The listing builds one solid part. Answer for the finished solid, in the listing's coordinates (mm). A direction names the side the tool comes from. Give positions to 0.01 mm unless a question says otherwise; leave off trailing zeros. Write each loop counter-clockwise with the first axis right and the second up, starting at its lowest first coordinate (ties: lowest second). Pieces come first, ordered by that corner, then holes. Notation, with made-up numbers: (11, 88) - (22, 88) arc R15 ccw to (22, 111) - close; hole circle Ø3 at (88.5, 18.5). An arc over 180 degrees is marked (long way). One line per question, with ' | ' between items. Start each with the question number.
1. Given P1, Ø3, axis at x = 0, y = 0, coming from the -Z side; P2, Ø1.5, axis at x = 10.5, z = 3.5, coming from the +Y side; P3, Ø2, axis at x = -1, z = 3, coming from the -Y side, each flat-ended and moving along its own axis, determine where each tip first touches the part or whether it passes through.
2. A cutting plane is placed at D-D (y = -7). Determine the outline of the cut face in (x, z).
3. A cutting plane is placed at A-A (x = 0). State how many separate pieces and enclosed holes the cut face has, then the cut area to 3 significant figures.
4. The mould has two halves that part along Y. Classify faces 4 (the face through (20.195, -2, 2)), 5 (the face through (28.13, 0, 1)), 6 (the face through (0, -26.618, 3)): +Y half, -Y half, draft (parallel to the pull), parting line (faces both ways), or undercut.
5. Find the intervals of material crossed by L1, parallel to Y at x = 0, z = 1.4 (1 decimal); L2, parallel to X at y = -14, z = 3.4, in increasing order. Write a range as from..to.
6. For faces 1 (the face through (-9.852, 10.015, 2.783)), 2 (the face through (2, 20.195, 2)), 3 (the face through (-26.618, 0, 3)), determine the directions among +Z, -Z, +X, -X, +Y, -Y from which every point of the face is accessible in a straight line to the end or side of a thin tool.
7. A cutting plane is placed at C-C (y = 19.5). Determine the outline of the cut face in (x, z).
Autodesk Inventor part; units mm, degrees
ref_plane "YZ Plane" through (0, 0, 0) normal (1, 0, 0) x (0, 1, 0)
ref_plane "XZ Plane" through (0, 0, 0) normal (0, 1, 0) x (-1, 0, 0)
ref_plane "XY Plane" through (0, 0, 0) normal (0, 0, 1) x (1, 0, 0)
sketch "Skizze1" plane through (0, 0, 0) normal (0, 0, 1) x (1, 0, 0)
  line L0 (-28.13, 28.13) -> (28.13, 28.13)
  line L1 (28.13, 28.13) -> (28.13, -28.13)
  line L2 (28.13, -28.13) -> (-28.13, -28.13)
  line L3 (-28.13, -28.13) -> (-28.13, 28.13)
  line L4 (-39.382, 0) -> (39.382, 0) construction
  line L5 (0, -39.382) -> (0, 39.382) construction
  point P0 (0, 0)
  dimension "d0" = 56.26
extrude "Extrusion1" add sketch "Skizze1" along normal blind 1.7
sketch "Skizze2" plane through (0, 0, 1.7) normal (0, 0, 1) x (1, 0, 0)
  line L0 (0, -39.382) -> (0, 39.382) construction
  line L1 (-39.382, 0) -> (39.382, 0) construction
  line L2 (-26.6175, 26.6175) -> (26.6175, 26.6175)
  line L3 (26.6175, 26.6175) -> (26.6175, -26.6175)
  line L4 (26.6175, -26.6175) -> (-26.6175, -26.6175)
  line L5 (-26.6175, -26.6175) -> (-26.6175, 26.6175)
  line L6 (28.13, 28.13) -> (-28.13, 28.13)
  point P0 (0, 0)
  dimension "d3" = 53.235
extrude "Extrusion2" add sketch "Skizze2" along normal blind 2.5
sketch "Skizze3" plane through (0, 0, 0) normal (0, 0, -1) x (-1, 0, 0)
  line L0 (28.13, -28.13) -> (-28.13, -28.13)
  line L1 (28.13, 28.13) -> (28.13, -28.13)
  line L2 (-28.13, 28.13) -> (28.13, 28.13)
  line L3 (-28.13, -28.13) -> (-28.13, 28.13)
  line L4 (-6.21, 20.195) -> (2.33, 20.195)
  line L5 (2.33, 20.195) -> (2.33, 7.76)
  line L6 (2.33, 7.76) -> (-6.21, 7.76)
  line L7 (-6.21, 7.76) -> (-6.21, 20.195)
  point P0 (0, 0)
  point P1 (0, 0)
  dimension "d6" = 21.92
  dimension "d7" = 8.54
  dimension "d8" = 12.435
  dimension "d9" = 35.89
extrude "Extrusion3" cut sketch "Skizze3" against normal up to surface (4.2 mm away) contours L4 L5 L6 L7
pattern_circular "Runde Anordnung1" count 4 over 360 about axis through (0, 0, -10) along (0, 0, 1) of "Extrusion3"
sketch "Skizze4" plane through (0, 0, 0) normal (0, 0, -1) x (-1, 0, 0)
  line L0 (-28.13, -28.13) -> (-28.13, 28.13)
  line L1 (-28.13, 28.13) -> (28.13, 28.13)
  point P0 (0, 0)
  point P1 (-11.817, 11.817)
  dimension "d15" = 16.313
  dimension "d16" = 16.313
hole "Bohrung1" at (11.817, 11.817, 0) direction (0, 0, 1) diameter 5.333 depth 3.35 counterbore diameter 8.2 counterbore depth 2.2
pattern_circular "Runde Anordnung2" count 4 over 360 about axis through (0, 0, -10) along (0, 0, 1) of "Bohrung1"
sketch "Skizze5" plane through (0, 0, 0) normal (0, 0, -1) x (-1, 0, 0)
  point P0 (0, 0)
  point P1 (0, 0)
hole "Bohrung2" at (0, 0, 0) direction (0, 0, 1) diameter 5.333 depth 3.35 counterbore diameter 11.199 counterbore depth 2.2
properties part number "PCB_cover_platte_originaldicke"
Determined:
1) P1: z = 3.35 | P2: y = 26.62 | P3: y = -26.62
2) outline: (-28.13, 0) - (28.13, 0) - (28.13, 1.7) - (26.62, 1.7) - (26.62, 4.2) - (-26.62, 4.2) - (-26.62, 1.7) - (-28.13, 1.7) - close
3) separate pieces: 3 | enclosed holes: 0 | area: 93.5 mm2
4) face 4: undercut | face 5: draft | face 6: -Y half
5) L1: -28.1..-20.2, -7.8..-5.6, 5.6..7.8, 20.2..28.1 | L2: -26.62..-6.21, 2.33..26.62
6) face 1: -Z | face 2: +Z, -Z | face 3: +Z, -X, +Y, -Y
7) outline: (-28.13, 0) - (-2.33, 0) - (-2.33, 4.2) - (-26.62, 4.2) - (-26.62, 1.7) - (-28.13, 1.7) - close; (6.21, 0) - (28.13, 0) - (28.13, 1.7) - (26.62, 1.7) - (26.62, 4.2) - (6.21, 4.2) - close
